```python
from build123d import *

# Parameters (mm, degrees)
SKETCH_W     = 100
SKETCH_H     = 100
PAD_DEPTH    = 50
SKETCH001_R  = 25
POCKET_DEPTH = 12.5
FILLET_R     = 20
FILLET001_R  = 2.5


with BuildPart() as part:
    # Sketch → Pad (new body)
    with BuildSketch(Plane.XY):
        Rectangle(SKETCH_W, SKETCH_H)
    extrude(amount=PAD_DEPTH)

    # Sketch001 (on Face6 of Pad) → Pocket (cut)
    with BuildSketch(Plane.XY.offset(50)):
        Circle(SKETCH001_R)
    extrude(amount=-POCKET_DEPTH, mode=Mode.SUBTRACT)

    # Fillet
    fillet_edges = [part.edges().sort_by_distance(p)[0] for p in [
        (50, -50, 25),
        (50, 50, 25),
        (-50, 50, 25),
        (-50, -50, 25),
    ]]
    fillet(fillet_edges, radius=FILLET_R)

    # Fillet001
    fillet001_edges = [part.edges().sort_by_distance(p)[0] for p in [
        (-25, 0, 50),
    ]]
    fillet(fillet001_edges, radius=FILLET001_R)


solid = part.part
```
Check sheet for the modelled part. Datum: model origin and axes. Units: mm. A direction names the side the tool comes from. Round coordinates to 2 decimals unless told otherwise and drop trailing zeros. Order: outer loops, then holes, each group sorted by start corner. A loop starts at its lowest first (then second) coordinate and runs counter-clockwise, first axis right, second up. Notation, with made-up numbers: (39.5, 14.25) - (47.5, 14.25) arc R19 ccw to (47.5, 22.25) - close; hole circle Ø8 at (38.5, -31). An arc over 180 degrees is marked (long way). Write item = value, one per line.
Q1. Section check A-A (y = 0). Record the boundary of the cut face in (x, z), and give its area (3 significant figures).
Computed:
outline = (-50, 0) - (50, 0) - (50, 50) - (27.5, 50) arc R2.5 ccw to (25, 47.5) - (25, 37.5) - (-25, 37.5) - (-25, 47.5) arc R2.5 ccw to (-27.5, 50) - (-50, 50) - close
area = 4,370 mm^2
Q2. Go/stop test with flat-tipped pins: pin 1 (5 mm diameter, centred on y = 36, z = 8, fed in from -X); pin 2 (1 mm diameter, centred on x = 8, y = -14.5, fed in from +Z). Record where each tip stops, or that it passes through.
Computed:
pin_1 = -49.69
pin_2 = 37.5
Q3. Draft check along Y on faces 3 (the face through (23.846, 7.509, 42.57)), 4 (the face through (0, 50, 25)), 5 (the face through (50, 0, 25)). Enter one of: pulls with the +Y half, pulls with the -Y half, needs draft (parallel to the pull), parting line crosses it, or undercut.
Computed:
face_3 = undercut
face_4 = pulls with the +Y half
face_5 = needs draft
Q4. Section check C-C (z = 27). Record the boundary of the cut face in (x, y), and give its area (3 significant figures).
Computed:
outline = (-50, -30) arc R20 ccw to (-30, -50) - (30, -50) arc R20 ccw to (50, -30) - (50, 30) arc R20 ccw to (30, 50) - (-30, 50) arc R20 ccw to (-50, 30) - close
area = 9,660 mm^2
Q5. Thickness scan on line 1 along Y through (x, z) = (0, 43); line 2 along Z through (x, y) = (5.5, -13); line 3 along X through (y, z) = (-11.5, 48). Record the ranges inside material, lowest first.
Computed:
line_1 = -50 to -25, 25 to 50
line_2 = 0 to 37.5
line_3 = -50 to -22.25, 22.25 to 50
Q6. Section check D-D (x = -36). Record the boundary of the cut face in (y, z).
Computed:
outline = (-49.08, 0) - (49.08, 0) - (49.08, 50) - (-49.08, 50) - close
Q7. Tool access check on faces 1 (the face through (0, 0, 37.5)), 2 (the face through (-50, 0, 25)). Record the directions out of +Z, -Z, +X, -X, +Y, -Y that give a thin tool (end or side, any length) a straight path to the whole face; none if there is none.
Computed:
face_1 = +Z
face_2 = +Z, -Z, -X, +Y, -Y
